from build123d import *

# Parameters (mm, degrees)
SKETCH_1_R          = 1.6
SKETCH_1_W          = 3.4
SKETCH_1_H          = 7.2
EXTRUDE_1_DEPTH     = 6
SKETCH_1_3_R        = 1.6
CUT_EXTRUDE_1_DEPTH = 4.5
SKETCH_2_R          = 2.1
CUT_EXTRUDE_2_DEPTH = 28.586228448
FILLET_1_R          = 1


with BuildPart() as part:
    # Sketch 1 → Extrude 1 (new, symmetric)
    # profile 1 of 2: a face of its own
    with BuildSketch(Plane.XY):
        with BuildLine():
            ThreePointArc((2.18016654, -7.697199092), (1.337547263, -8.987840658), (2.5, -10))
            ThreePointArc((2.5, -10), (0.263932023, -9.472135955), (-1.5, -8))
            Line((-1.5, -8), (-4.8, -3.6))
            ThreePointArc((-4.8, -3.6), (-6, 0), (-4.8, 3.6))
            Line((-4.8, 3.6), (-1.5, 8))
            ThreePointArc((-1.5, 8), (0.263932023, 9.472135955), (2.5, 10))
            ThreePointArc((2.5, 10), (1.337547263, 8.987840658), (2.18016654, 7.697199092))
            ThreePointArc((2.18016654, 7.697199092), (8, 0), (2.18016654, -7.697199092))
        make_face()
        Circle(SKETCH_1_R, mode=Mode.SUBTRACT)
    # profile 2 of 2: a face of its own
    with BuildSketch(Plane.XY):
        with BuildLine():
            ThreePointArc((2.18016654, -7.697199092), (8, 0), (2.18016654, 7.697199092))
            ThreePointArc((2.18016654, 7.697199092), (1.337547263, 8.987840658), (2.5, 10))
            Line((2.5, 10), (19, 10))
            Line((19, 10), (19, -10))
            Line((19, -10), (2.5, -10))
            ThreePointArc((2.5, -10), (1.337547263, -8.987840658), (2.18016654, -7.697199092))
        make_face()
        with Locations((14.3, 0)):
            Rectangle(SKETCH_1_W, SKETCH_1_H, mode=Mode.SUBTRACT)
    extrude(amount=EXTRUDE_1_DEPTH, both=True)

    # Sketch 1_3 → Cut-Extrude 1 (cut, symmetric)
    with BuildSketch(Plane.XY):
        with BuildLine():
            ThreePointArc((2.18016654, -7.697199092), (1.337547263, -8.987840658), (2.5, -10))
            ThreePointArc((2.5, -10), (0.263932023, -9.472135955), (-1.5, -8))
            Line((-1.5, -8), (-4.8, -3.6))
            ThreePointArc((-4.8, -3.6), (-6, 0), (-4.8, 3.6))
            Line((-4.8, 3.6), (-1.5, 8))
            ThreePointArc((-1.5, 8), (0.263932023, 9.472135955), (2.5, 10))
            ThreePointArc((2.5, 10), (1.337547263, 8.987840658), (2.18016654, 7.697199092))
            ThreePointArc((2.18016654, 7.697199092), (8, 0), (2.18016654, -7.697199092))
        make_face()
        Circle(SKETCH_1_3_R, mode=Mode.SUBTRACT)
    extrude(amount=CUT_EXTRUDE_1_DEPTH, both=True, mode=Mode.SUBTRACT)

    # Sketch 2 → Cut-Extrude 2 (cut, through all)
    with BuildSketch(Plane(origin=(19, 0, 0), x_dir=(0, 0, -1), z_dir=(1, 0, 0))):
        Circle(SKETCH_2_R)
    extrude(amount=-CUT_EXTRUDE_2_DEPTH, mode=Mode.SUBTRACT)

    # Fillet 1
    fillet_1_edges = [part.edges().sort_by_distance(p)[0] for p in [
        (7.999999993, 1e-09, 2.100000016),
        (19, 0, 2.1),
    ]]
    fillet(fillet_1_edges, radius=FILLET_1_R)


solid = part.part
The listing builds one solid part. Answer for the finished solid, in the listing's coordinates (mm). A direction names the side the tool comes from. Round coordinates to 2 decimals unless told otherwise and drop trailing zeros. Order: outer loops, then holes, each group sorted by start corner. A loop starts at its lowest first (then second) coordinate and runs counter-clockwise, first axis right, second up. Notation, with made-up numbers: M 12.25,-9 L 48.25,-9 A7 cw 48.25,-3 Z; hole C 49,44 d2. An arc over 180 degrees is marked long. Answer in a Markdown table with one row per item. Add a question column.
1) The part is cut by section A-A on x = 15.25. Determine the outline of the cut face in (y, z).
2) The part is cut by section C-C on y = 0. Count the separate pieces of the cut face and the enclosed holes in it, plus the area to 3 significant figures.
3) The part is cut by section D-D on y = -4.25. Determine the outline of the cut face in (x, z).
4) Flat-ended cylindrical pins translate along their axes: pin 1 Ø1.5 at (x, z) = (1, -2.5) entering from +Y; pin 2 Ø6 at (y, z) = (0.5, -1) entering from -X; pin 3 Ø4 at (y, z) = (0, 0) entering from -X; pin 4 Ø5.5 at (y, z) = (0, 0) entering from -X. Find the tip coordinate at first contact, or state that the pin passes through.
5) Determine the mould class of faces 4 (the face through (0.235, 9.458, -5.24)), 5 (the face through (7, 0, -6)), 6 (the face through (3, 0, 4.5)) for opening direction Y: pulls with the +Y half, pulls with the -Y half, needs draft (parallel to the pull), parting line crosses it, or undercut.
6) Which of the six approach directions +Z, -Z, +X, -X, +Y, -Y give full straight-line access (tool end or side, diameter ignored) to faces 1 (the face through (16, 2.3, 0.1)), 2 (the face through (7.63, 2.41, 2.06)), 3 (the face through (17.014, 0.631, -2.003))?
7) Consider line 1 along Z through (x, y) = (5.25, -1.25); line 2 along Y through (x, z) = (17.4, 0); line 3 along Y through (x, z) = (5.5, 2.25). Determine where each line is inside the solid, lowest interval first. Write a range as from..to.
8) The part is cut by section B-B on x = 3.75. Determine the outline of the cut face in (y, z), plus the area to 3 significant figures.
Findings below:
| question | item | result |
|---|---|---|
| 1 | outline | M -10,-6 L -3.6,-6 L -3.6,6 L -10,6 Z; M 3.6,-6 L 10,-6 L 10,6 L 3.6,6 Z |
| 2 | separate pieces | 6 |
| 2 | enclosed holes | 0 |
| 2 | area | 90.8 mm² |
| 3 | outline | M -4.31,-6 L 19,-6 L 19,6 L -4.31,6 L -4.31,4.5 L 6.78,4.5 L 6.78,-4.5 L -4.31,-4.5 Z |
| 4 | pin 1 | stops at y = 9.73 |
| 4 | pin 2 | stops at x = 7.19 |
| 4 | pin 3 | passes through |
| 4 | pin 4 | stops at x = 7.51 |
| 5 | face 4 | pulls with the +Y half |
| 5 | face 5 | needs draft |
| 5 | face 6 | undercut |
| 6 | face 1 | +Z, -Z |
| 6 | face 2 | -X |
| 6 | face 3 | +X, -X |
| 7 | line 1 | z = -6..-4.5, 4.5..6 |
| 7 | line 2 | y = -10..-2.1, 2.1..10 |
| 7 | line 3 | y = -10..-5.81, 5.81..10 |
| 8 | outline | M -10,-6 L 10,-6 L 10,6 L -10,6 Z; hole M -7.07,-4.5 L 7.07,-4.5 L 7.07,4.5 L -7.07,4.5 Z |
| 8 | area | 113 mm² |
